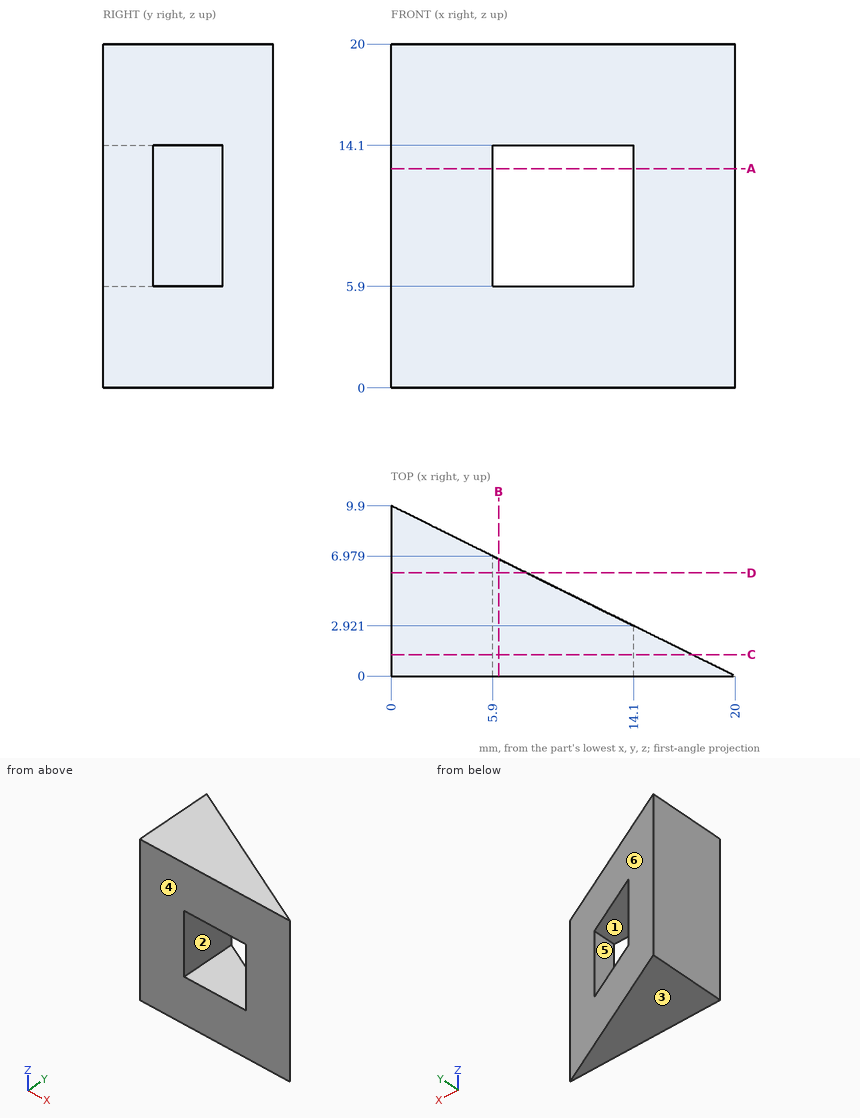
The figure shows three views and two pictorial views of one solid part (mm, origin at its lowest corner). Answer the questions. A direction names the side the tool comes from. Round coordinates to 2 decimals unless told otherwise and drop trailing zeros. Write each loop counter-clockwise with the first axis right and the second up, starting at its lowest first coordinate (ties: lowest second). Pieces come first, ordered by that corner, then holes. Notation, with made-up numbers: (-25.5, 88) -> (7.5, 88) arc R25 cw to (7.5, 115) -> close; hole circle Ø7 at (42.25, 16.5). An arc over 180 degrees is marked (long way). Answer as a JSON object with one key per item and string values. Group by question number.
Q1. Section A-A (z = 12.75) is taken. Write down the section's boundary in (x, y).
Q2. Section D-D (y = 6) is taken. Write down the section's boundary in (x, z), plus the area to 3 significant figures.
Q3. Section B-B (x = 6.25) is taken. Write down the section's boundary in (y, z).
Q4. Each of these flat-tipped pins is pushed along its axis until it touches: pin 1 Ø5.5 at (x, y) = (11, 5) entering from -Z; pin 2 Ø1.5 at (x, z) = (12, 18) entering from +Y; pin 3 Ø2 at (x, z) = (6.5, 3.5) entering from +Y; pin 4 Ø5.5 at (y, z) = (3, 11) entering from +X (1 decimal). Where does it stop, or does it pass through?
Q5. Which of the six approach directions +Z, -Z, +X, -X, +Y, -Y give full straight-line access (tool end or side, diameter ignored) to the marked faces 5 and 6?
Q6. Section C-C (y = 1.25) is taken. Write down the section's boundary in (x, z) (1 decimal), plus the area to 3 significant figures.
Q7. Straight lines are drawn through the part: line 1 along X through (y, z) = (3.25, 6.25); line 2 along Z through (x, y) = (8, 2); line 3 along X through (y, z) = (2, 8.5) (1 decimal). For each, find the intervals that lie inside material, in ascending order.
Q8. Determine the mould class of the marked faces 1, 2, 3 and 4 for opening direction Z: pulls with the +Z half, pulls with the -Z half, needs draft (parallel to the pull), parting line crosses it, or undercut.
Check values:
{
 "1": {"outline": "(0, 0) -> (5.9, 0) -> (5.9, 6.98) -> (0, 9.9) -> close; (14.1, 0) -> (20, 0) -> (14.1, 2.92) -> close"},
 "2": {"outline": "(0, 0) -> (7.88, 0) -> (7.88, 5.9) -> (5.9, 5.9) -> (5.9, 14.1) -> (7.88, 14.1) -> (7.88, 20) -> (0, 20) -> close", "area": "141 mm^2"},
 "3": {"outline": "(0, 0) -> (6.81, 0) -> (6.81, 5.9) -> (0, 5.9) -> close; (0, 14.1) -> (6.81, 14.1) -> (6.81, 20) -> (0, 20) -> close"},
 "4": {"pin 1": "z = 0", "pin 2": "y = 4.33", "pin 3": "y = 7.18", "pin 4": "x = 19.5"},
 "5": {"face 5": "+Y, -Y", "face 6": "+Z, -Z, +X, +Y"},
 "6": {"outline": "(0, 0) -> (17.5, 0) -> (17.5, 20) -> (0, 20) -> close; hole (5.9, 5.9) -> (14.1, 5.9) -> (14.1, 14.1) -> (5.9, 14.1) -> close", "area": "282 mm^2"},
 "7": {"line 1": "0 to 5.9", "line 2": "0 to 5.9, 14.1 to 20", "line 3": "0 to 5.9, 14.1 to 16"},
 "8": {"face 1": "undercut", "face 2": "undercut", "face 3": "pulls with the -Z half", "face 4": "needs draft"}
}
